```python
from build123d import *

# Parameters (mm, degrees)
CUT_EXTRUDE5_DEPTH = 62.806608676
CUT_EXTRUDE6_DEPTH = 2.54
CIRPATTERN1_COUNT  = 5
CIRPATTERN2_COUNT  = 8


with BuildPart() as part:
    # Sketch1 → Revolve1 (revolve)
    with BuildSketch(Plane(origin=(0, 0, 0), x_dir=(0, 0, -1), z_dir=(1, 0, 0)), mode=Mode.PRIVATE) as revolve1_sk:
        with BuildLine():
            Line((0, 12.7), (0, 10.16))
            Line((0, 10.16), (10.16, 10.16))
            Line((10.16, 10.16), (10.16, 35.052))
            Line((10.16, 35.052), (21.59, 38.1))
            Line((21.59, 38.1), (21.59, 41.91))
            Line((21.59, 41.91), (-6.35, 41.91))
            Line((-6.35, 41.91), (-6.35, 38.1))
            Line((-6.35, 38.1), (-1.016, 38.1))
            ThreePointArc((-1.016, 38.1), (2.576102448, 36.612102448), (4.064, 33.02))
            Line((4.064, 33.02), (4.064, 12.7))
            Line((4.064, 12.7), (0, 12.7))
        make_face()
    revolve(revolve1_sk.sketch.rotate(Axis((0, 0, 0), (0, 0, -1)), 90), axis=Axis((0, 0, 0), (0, 0, -1)))

    # Sketch2 → Cut-Extrude5 (cut, through all)
    with BuildSketch(Plane.XY.offset(-4.064)):
        with BuildLine():
            Line((-7.888804495, 29.441419185), (-6.245303558, 23.307790188))
            ThreePointArc((-6.245303558, 23.307790188), (0, 24.13), (6.245303558, 23.307790188))
            Line((6.245303558, 23.307790188), (7.888804495, 29.441419185))
            ThreePointArc((7.888804495, 29.441419185), (0, 30.48), (-7.888804495, 29.441419185))
        make_face()
    cut_extrude5 = extrude(amount=-CUT_EXTRUDE5_DEPTH, mode=Mode.SUBTRACT)

    # Sketch2_9 → Cut-Extrude6 (cut)
    with BuildSketch(Plane.XY.offset(-4.064)):
        with BuildLine():
            Line((2.032, 20.32), (2.032, 15.24))
            ThreePointArc((2.032, 15.24), (0, 13.208), (-2.032, 15.24))
            Line((-2.032, 15.24), (-2.032, 20.32))
            ThreePointArc((-2.032, 20.32), (0, 22.352), (2.032, 20.32))
        make_face()
    cut_extrude6 = extrude(amount=-CUT_EXTRUDE6_DEPTH, mode=Mode.SUBTRACT)

    # CirPattern1: Cut-Extrude6 ×5 about axis
    cirpattern1_axis = Axis((0, 0, 0), (0, 0, 1))
    for i in range(1, CIRPATTERN1_COUNT):
        add(cut_extrude6.rotate(cirpattern1_axis, i * 360 / CIRPATTERN1_COUNT), mode=Mode.SUBTRACT)

    # CirPattern2: Cut-Extrude5 ×8 about axis, 1 skipped
    cirpattern2_axis = Axis((0, 0, 0), (0, 0, 1))
    add([cut_extrude5.rotate(cirpattern2_axis, i * 360 / CIRPATTERN2_COUNT) for i in range(1, CIRPATTERN2_COUNT) if i not in (4,)], mode=Mode.SUBTRACT)


solid = part.part
```
Can you work these out from the model? Positions are in its coordinate system, mm. A direction names the side the tool comes from. Coordinates: 2 decimals unless noted, no trailing zeros. Order: outer loops, then holes, each group sorted by start corner. A loop starts at its lowest first (then second) coordinate and runs counter-clockwise, first axis right, second up. Notation, with made-up numbers: (28.5, 14) -> (33.5, 14) arc R22 ccw to (33.5, 25) -> close; hole circle Ø1 at (59, 35.25). An arc over 180 degrees is marked (long way). Write each question's results on one line, items separated by ' | '.
Item 1: I want a section at C-C, the plane z = -1. Write out the boundary of the cut face in (x, y), then the cut area to 3 significant figures.
Results are:
outline: circle Ø83.82 at (0, 0); circle Ø25.4 at (0, 0); hole circle Ø75.37 at (0, 0); hole circle Ø20.32 at (0, 0) | area: 1,240 mm²
Item 2: I want a section at D-D, the plane z = 4.75. Write out the boundary of the cut face in (x, y).
Results are:
outline: circle Ø83.82 at (0, 0); hole circle Ø76.2 at (0, 0)
Item 3: I'm going to push flat-ended pins straight in: pin 1 Ø1.7 at (x, y) = (17, 6.5) entering from +Z; pin 2 Ø2 at (y, z) = (17.5, -5) entering from -X; pin 3 Ø5 at (y, z) = (-8, -3.5) entering from +X. Where does each tip first touch, or does it pass through?
Results are:
pin 1: z = -6.6 | pin 2: x = -38.53 | pin 3: x = 41.55
Item 4: If I drill on line 1 along Y through (x, z) = (0, -8); line 2 along Y through (x, z) = (0, -5.5); line 3 along Y through (x, z) = (-21.5, -6.25), over which ranges is the centre line in solid material (lowest first)?
Results are:
line 1: -41.91 to -10.16, 10.16 to 24.13, 30.48 to 41.91 | line 2: -41.91 to -10.16, 10.16 to 13.21, 22.35 to 24.13, 30.48 to 41.91 | line 3: -35.97 to -21.61, -12.41 to 12.41, 21.61 to 35.97
Item 5: If we mould it in two halves opening along X, with no side actions, what happens to faces 1 (the face through (-5.456, -41.553, -7.424)), 2 (the face through (-13.63, 23.61, -7.07)), 3 (the face through (-10, 37, 6.35))? For each: +X half, -X half, draft (parallel to the pull), parting line (faces both ways), or undercut.
Results are:
face 1: parting line | face 2: undercut | face 3: draft
Item 6: Which directions (+Z, -Z, +X, -X, +Y, -Y) give clear straight access to the entire face, cutting with the end or side of a thin tool? Please do faces 4 (the face through (16.26, 31.27, -10.88)), 5 (the face through (13.63, -23.61, -7.07)), 6 (the face through (10, -14, -6.604)).
Results are:
face 4: -Z | face 5: +Z, -Z | face 6: +Z
Item 7: I want a section at A-A, the plane x = 0. Count the separate pieces of the cut face and the enclosed holes in it, then the cut area to 3 significant figures.
Results are:
separate pieces: 3 | enclosed holes: 0 | area: 558 mm²
